Can you work these out from the model? Positions are in its coordinate system, mm. Give positions to 0.01 mm unless a question says otherwise; leave off trailing zeros. Loops run counter-clockwise (first coordinate to the right, second up) from the corner with the lowest first, then second, coordinate; pieces in that order, holes last. Notation, with made-up numbers: (-33.5, 73.25) -> (22.5, 73.25) arc R16 ccw to (22.5, 98.25) -> close; hole circle Ø1 at (77.25, 19). An arc over 180 degrees is marked (long way). One line per question, with ' | ' between items.
from build123d import *

# Parameters (mm, degrees)
SKETCH1_R           = 2
SKETCH1_R_2         = 2.5
BOSS_EXTRUDE1_DEPTH = 4
SKETCH2_W           = 1
SKETCH2_H           = 25
CUT_EXTRUDE1_DEPTH  = 1


with BuildPart() as part:
    # Sketch1 → Boss-Extrude1 (new body)
    with BuildSketch(Plane(origin=(0, 0, 0), x_dir=(1, 0, 0), z_dir=(0, 1, 0))):
        with BuildLine():
            Line((25.625, 28.625), (-25.625, 28.625))
            ThreePointArc((-25.625, 28.625), (-27.746320344, 27.746320344), (-28.625, 25.625))
            Line((-28.625, 25.625), (-28.625, -25.625))
            ThreePointArc((-28.625, -25.625), (-27.746320344, -27.746320344), (-25.625, -28.625))
            Line((-25.625, -28.625), (25.625, -28.625))
            ThreePointArc((25.625, -28.625), (27.746320344, -27.746320344), (28.625, -25.625))
            Line((28.625, -25.625), (28.625, 25.625))
            ThreePointArc((28.625, 25.625), (27.746320344, 27.746320344), (25.625, 28.625))
        make_face()
        with Locations(Location((-15.5, 15.5, 0), (0, 0, 270))):
            Circle(SKETCH1_R, mode=Mode.SUBTRACT)
        with Locations(Location((-23.57, 23.57, 0), (0, 0, 270))):
            Circle(SKETCH1_R_2, mode=Mode.SUBTRACT)
        with Locations(Location((23.57, 23.57, 0), (0, 0, 270))):
            Circle(SKETCH1_R_2, mode=Mode.SUBTRACT)
        with Locations(Location((15.5, 15.5, 0), (0, 0, 270))):
            Circle(SKETCH1_R, mode=Mode.SUBTRACT)
        with Locations(Location((15.5, -15.5, 0), (0, 0, 270))):
            Circle(SKETCH1_R, mode=Mode.SUBTRACT)
        with Locations(Location((-15.5, -15.5, 0), (0, 0, 270))):
            Circle(SKETCH1_R, mode=Mode.SUBTRACT)
        with Locations(Location((-23.57, -23.57, 0), (0, 0, 270))):
            Circle(SKETCH1_R_2, mode=Mode.SUBTRACT)
        with Locations(Location((23.57, -23.57, 0), (0, 0, 270))):
            Circle(SKETCH1_R_2, mode=Mode.SUBTRACT)
    extrude(amount=BOSS_EXTRUDE1_DEPTH)

    # Sketch2 → Cut-Extrude1 (cut)
    with BuildSketch(Plane(origin=(0, 4, 0), x_dir=(1, 0, 0), z_dir=(0, 1, 0))):
        with Locations((-27.125, 0)):
            Rectangle(SKETCH2_W, SKETCH2_H)
        with Locations((-25.125, 0)):
            Rectangle(SKETCH2_W, SKETCH2_H)
        with Locations((-23.125, 0)):
            Rectangle(SKETCH2_W, SKETCH2_H)
        with Locations((-21.125, 0)):
            Rectangle(SKETCH2_W, SKETCH2_H)
        with Locations((-19.125, 0)):
            Rectangle(SKETCH2_W, SKETCH2_H)
        with Locations((-17.125, 0)):
            Rectangle(SKETCH2_W, SKETCH2_H)
        with Locations((-15.125, 0)):
            Rectangle(SKETCH2_W, SKETCH2_H)
        with Locations((-13.125, 0)):
            Rectangle(SKETCH2_W, SKETCH2_H)
        with Locations((-11.125, 0)):
            Rectangle(SKETCH2_W, SKETCH2_H)
        with Locations((-9.125, 0)):
            Rectangle(SKETCH2_W, SKETCH2_H)
        with Locations((-7.125, 0)):
            Rectangle(SKETCH2_W, SKETCH2_H)
        with Locations((-5.125, 0)):
            Rectangle(SKETCH2_W, SKETCH2_H)
        with Locations((-3.125, 0)):
            Rectangle(SKETCH2_W, SKETCH2_H)
        with Locations((-1.125, 0)):
            Rectangle(SKETCH2_W, SKETCH2_H)
        with Locations((0.875, 0)):
            Rectangle(SKETCH2_W, SKETCH2_H)
        with Locations((2.875, 0)):
            Rectangle(SKETCH2_W, SKETCH2_H)
        with Locations((4.875, 0)):
            Rectangle(SKETCH2_W, SKETCH2_H)
        with Locations((6.875, 0)):
            Rectangle(SKETCH2_W, SKETCH2_H)
        with Locations((8.875, 0)):
            Rectangle(SKETCH2_W, SKETCH2_H)
        with Locations((10.875, 0)):
            Rectangle(SKETCH2_W, SKETCH2_H)
        with Locations((12.875, 0)):
            Rectangle(SKETCH2_W, SKETCH2_H)
        with Locations((14.875, 0)):
            Rectangle(SKETCH2_W, SKETCH2_H)
        with Locations((16.875, 0)):
            Rectangle(SKETCH2_W, SKETCH2_H)
        with Locations((18.875, 0)):
            Rectangle(SKETCH2_W, SKETCH2_H)
        with Locations((20.875, 0)):
            Rectangle(SKETCH2_W, SKETCH2_H)
        with Locations((22.875, 0)):
            Rectangle(SKETCH2_W, SKETCH2_H)
        with Locations((24.875, 0)):
            Rectangle(SKETCH2_W, SKETCH2_H)
        with Locations((26.875, 0)):
            Rectangle(SKETCH2_W, SKETCH2_H)
    extrude(amount=-CUT_EXTRUDE1_DEPTH, mode=Mode.SUBTRACT)


solid = part.part
Q1. If we mould it in two halves opening along Z, with no side actions, what happens to faces 1 (the face through (0, 0, 0)), 2 (the face through (-27.72, 1.97, -27.77)), 3 (the face through (-13.517, 1.972, 15.24))? For each: pulls with the +Z half, pulls with the -Z half, needs draft (parallel to the pull), parting line crosses it, or undercut.
Entries:
face 1: needs draft | face 2: pulls with the -Z half | face 3: undercut
Q2. If we section it at B-B (y = 1.5): State how many separate pieces and enclosed holes the cut face has, plus the area to 3 significant figures.
Entries:
separate pieces: 1 | enclosed holes: 8 | area: 3,140 mm²
Q3. If I drill on probe 1 along X at (y, z) = (2.45, 23.57) (3 decimals); probe 2 along Z at (x, y) = (-13, 3.45) (3 decimals); probe 3 along Z at (x, y) = (16.5, 2.3) (3 decimals), over which ranges is the centre line in solid material (lowest first)? Write a range as from..to.
Entries:
probe 1: -28.625..-26.07, -21.07..21.07, 26.07..28.625 | probe 2: -28.625..-12.5, 12.5..28.625 | probe 3: -28.625..-17.232, -13.768..13.768, 17.232..28.625
Q4. If we section it at A-A (z = -23.57): Write out the boundary of the cut face in (x, y) (3 decimals).
Entries:
outline: (-28.625, 0) -> (-26.07, 0) -> (-26.07, 4) -> (-28.625, 4) -> close; (-21.07, 0) -> (21.07, 0) -> (21.07, 4) -> (-21.07, 4) -> close; (26.07, 0) -> (28.625, 0) -> (28.625, 4) -> (26.07, 4) -> close
Q5. If we section it at C-C (z = -15.5): Write out the boundary of the cut face in (x, y) (3 decimals).
Entries:
outline: (-28.625, 0) -> (-17.5, 0) -> (-17.5, 4) -> (-28.625, 4) -> close; (-13.5, 0) -> (13.5, 0) -> (13.5, 4) -> (-13.5, 4) -> close; (17.5, 0) -> (28.625, 0) -> (28.625, 4) -> (17.5, 4) -> close
